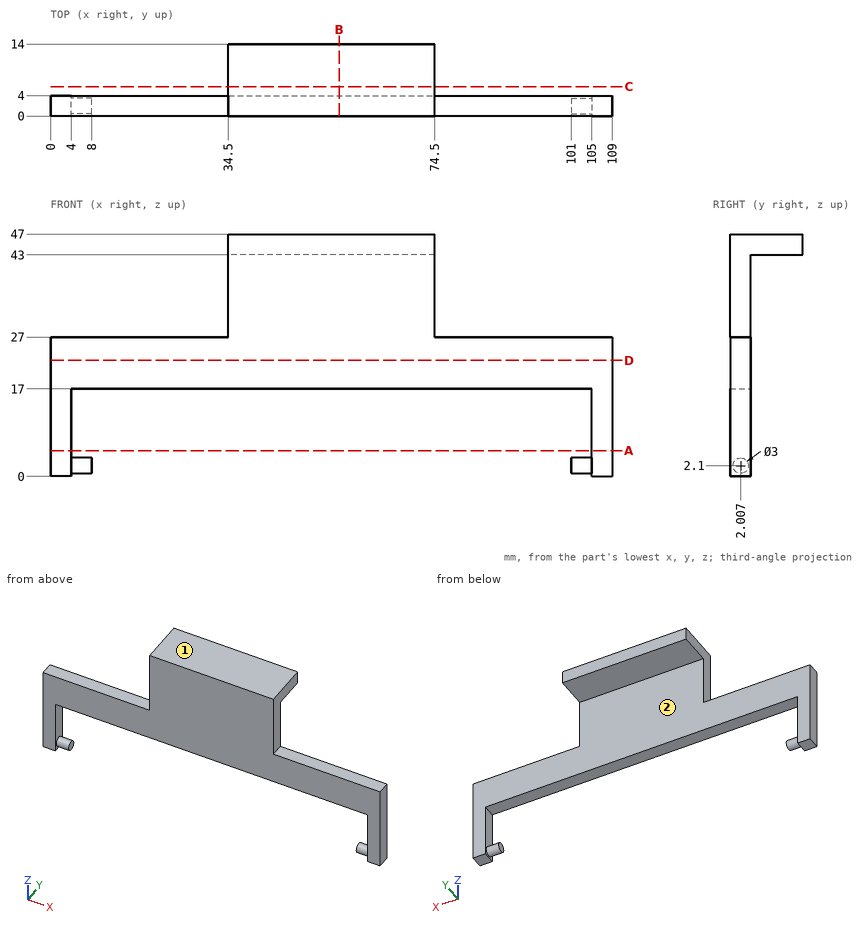
For this review, use the dimensioned drawing (mm, ordinates from the lowest corner) and the shaded views. A direction names the side the tool comes from. Coordinates: 2 decimals unless noted, no trailing zeros. Order: outer loops, then holes, each group sorted by start corner. A loop starts at its lowest first (then second) coordinate and runs counter-clockwise, first axis right, second up. Notation, with made-up numbers: (87, -38) - (141, -38) arc R17 cw to (141, -16) - close; hole circle Ø7 at (-40, 55). An arc over 180 degrees is marked (long way). Answer in a Markdown table with one row per item.
(1) Clearance check with flat-ended pins moving along their axes: pin 1 (1.2 mm diameter, centred on x = 87, y = 2.5, fed in from +Z); pin 2 (3 mm diameter, centred on x = 42, y = 2.5, fed in from -Z); pin 3 (5 mm diameter, centred on x = 53, z = 21.5, fed in from +Y); pin 4 (7 mm diameter, centred on y = 9, z = 35.5, fed in from +X). State where each tip first meets the part, or that it passes through.
Checked values:
| item | result |
|---|---|
| pin 1 | z = 27 |
| pin 2 | z = 17 |
| pin 3 | y = 4 |
| pin 4 | through |
(2) For the marked faces 1 and 2, list the 3-axis set-ups (+Z, -Z, +X, -X, +Y, -Y) from which the entire face can be reached by the end or side of a thin tool; tool diameter is ignored.
Checked values:
| item | result |
|---|---|
| face 1 | +Z, +X, -X, +Y, -Y |
| face 2 | -Z, +X, -X, +Y |
(3) Wall thickness on line 1 along X through (y, z) = (3.5, 8); line 2 along Z through (x, y) = (26, 1); line 3 along Z through (x, y) = (71, 6): over which ranges is each line inside the solid? List them lowest first. Write a range as from..to.
Checked values:
| item | result |
|---|---|
| line 1 | 0..4, 105..109 |
| line 2 | 17..27 |
| line 3 | 43..47 |
(4) Consider section B-B on x = 56. State the section outline as (y, z) points.
Checked values:
| item | result |
|---|---|
| outline | (0, 17) - (4, 17) - (4, 43) - (14, 43) - (14, 47) - (0, 47) - close |
(5) Consider section A-A on z = 5. State the section outline as (x, y) points.
Checked values:
| item | result |
|---|---|
| outline | (0, 0) - (4, 0) - (4, 4) - (0, 4) - close; (105, 0) - (109, 0) - (109, 4) - (105, 4) - close |
(6) Consider section D-D on z = 22.5. State the section outline as (x, y) points, plus the area to 3 significant figures.
Checked values:
| item | result |
|---|---|
| outline | (0, 0) - (109, 0) - (109, 4) - (0, 4) - close |
| area | 436 mm^2 |
(7) Consider section C-C on y = 5.75. State the section outline as (x, z) points, plus the area to 3 significant figures.
Checked values:
| item | result |
|---|---|
| outline | (34.5, 43) - (74.5, 43) - (74.5, 47) - (34.5, 47) - close |
| area | 160 mm^2 |
